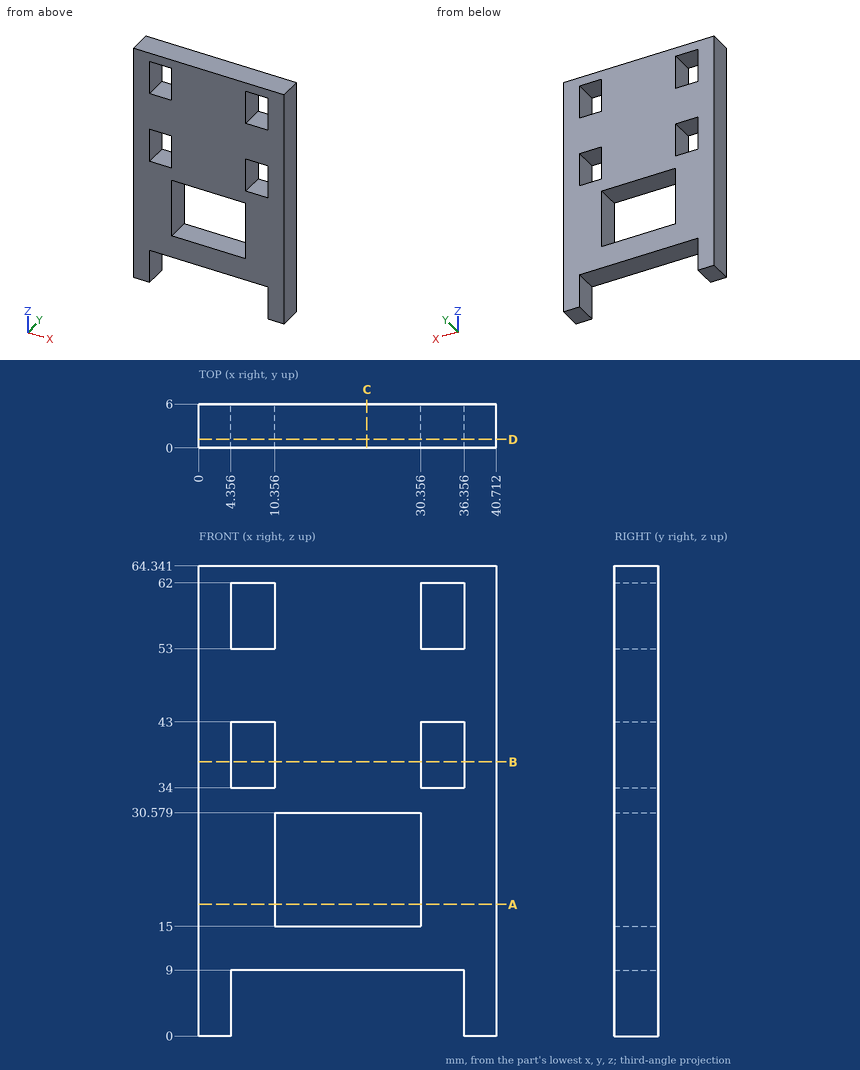
Source: three-view drawing plus pictorial views. Frame: mm from the lowest corner of the part. Coordinates: 2 decimals unless noted, no trailing zeros. Write each loop counter-clockwise with the first axis right and the second up, starting at its lowest first coordinate (ties: lowest second). Pieces come first, ordered by that corner, then holes. Notation, with made-up numbers: (67, 7.5) -> (121, 7.5) arc R13 ccw to (121, 13.5) -> close; hole circle Ø10 at (41.5, 32). An arc over 180 degrees is marked (long way). Write each question's results on one line, items separated by ' | '.
Item 1: Section query A-A on z = 18. Return loops of the section in (x, y).
Conclusion:
outline: (0, 0) -> (10.36, 0) -> (10.36, 6) -> (0, 6) -> close; (30.36, 0) -> (40.71, 0) -> (40.71, 6) -> (30.36, 6) -> close
Item 2: Pin query (flat end, axial travel): pin 1 Ø1 at (x, z) = (34, 36.5) entering from +Y; pin 2 Ø3 at (x, y) = (19, 2.5) entering from -Z. Return the tip coordinate at first contact, or that it passes through.
Conclusion:
pin 1: passes through | pin 2: stops at z = 9
Item 3: Material intervals for probe 1 along Z at (x, y) = (5, 4.1); probe 2 along X at (y, z) = (3.55, 57.5); probe 3 along Z at (x, y) = (29.5, 2), sorted ascending.
Conclusion:
probe 1: z = 9 to 34, 43 to 53, 62 to 64.34 | probe 2: x = 0 to 4.36, 10.36 to 30.36, 36.36 to 40.71 | probe 3: z = 9 to 15, 30.58 to 64.34
Item 4: Section query D-D on y = 1.15. Return loops of the section in (x, z), plus the area to 3 significant figures.
Conclusion:
outline: (0, 0) -> (4.36, 0) -> (4.36, 9) -> (36.36, 9) -> (36.36, 0) -> (40.71, 0) -> (40.71, 64.34) -> (0, 64.34) -> close; hole (4.36, 34) -> (10.36, 34) -> (10.36, 43) -> (4.36, 43) -> close; hole (4.36, 53) -> (10.36, 53) -> (10.36, 62) -> (4.36, 62) -> close; hole (10.36, 15) -> (30.36, 15) -> (30.36, 30.58) -> (10.36, 30.58) -> close; hole (30.36, 34) -> (36.36, 34) -> (36.36, 43) -> (30.36, 43) -> close; hole (30.36, 53) -> (36.36, 53) -> (36.36, 62) -> (30.36, 62) -> close | area: 1,800 mm^2
Item 5: Section query C-C on x = 23. Return loops of the section in (y, z), plus the area to 3 significant figures.
Conclusion:
outline: (0, 9) -> (6, 9) -> (6, 15) -> (0, 15) -> close; (0, 30.58) -> (6, 30.58) -> (6, 64.34) -> (0, 64.34) -> close | area: 239 mm^2
Item 6: Section query B-B on z = 37.5. Return loops of the section in (x, y), plus the area to 3 significant figures.
Conclusion:
outline: (0, 0) -> (4.36, 0) -> (4.36, 6) -> (0, 6) -> close; (10.36, 0) -> (30.36, 0) -> (30.36, 6) -> (10.36, 6) -> close; (36.36, 0) -> (40.71, 0) -> (40.71, 6) -> (36.36, 6) -> close | area: 172 mm^2
